Autodesk Fusion 360 part; units mm, degrees
sketch "Sketch1" plane through (0, 0, 0) normal (0, 1, 0) x (1, 0, 0)
  line L0 (0, 0) -> (250.5, 0) construction
  line L1 (250.5, 0) -> (250.5, -213.77) construction
  line L2 (250.5, -213.77) -> (0, -213.77) construction
  line L3 (0, -213.77) -> (0, 0) construction
  dimension "d1" = 250.5
  dimension "d2" = 213.77
sketch "Sketch2" plane through (0, 0, 0) normal (0, 1, 0) x (1, 0, 0)
  line L0 (0, 0) -> (250, 0) construction
  line L1 (250, 0) -> (250, -129.65) construction
  line L2 (250, -129.65) -> (0, -129.65) construction
  line L3 (0, -129.65) -> (0, 0) construction
  line L4 (193.51, 174.3203) -> (193.51, 171.7713)
  line L5 (193.51, -171.7713) -> (193.51, -174.3361)
  line L6 (169.51, 168.436) -> (169.51, 165.8296)
  line L7 (169.51, -165.8296) -> (169.51, -168.436)
  line L8 (133.51, 155.0829) -> (133.51, 152.3361)
  line L9 (133.51, -152.3361) -> (133.51, -155.0829)
  line L10 (110.01, 143.0564) -> (110.01, 140.1696)
  line L11 (110.01, -140.1696) -> (110.01, -143.0564)
  line L12 (228.8785, 178.9674) -> (228.8785, -179.12)
  arc A0 (193.51, 171.7713) -> (169.51, 165.8296) centre (246.9617, -95.5777) ccw
  arc A1 (169.51, -165.8296) -> (193.51, -171.7713) centre (246.9617, 95.5777) ccw
  arc A2 (133.51, 152.3361) -> (110.01, 140.1696) centre (246.9617, -95.5777) ccw
  arc A3 (110.01, -140.1696) -> (133.51, -152.3361) centre (246.9617, 95.5777) ccw
  arc A4 (228.8785, 178.9674) -> (193.51, 174.3203) centre (246.9617, -95.5777) ccw
  arc A5 (193.51, -174.3361) -> (228.8785, -179.12) centre (247.9959, 95.355) ccw
  arc A6 (169.51, 168.436) -> (133.51, 155.0829) centre (246.9617, -95.5777) ccw
  arc A7 (133.51, -155.0829) -> (169.51, -168.436) centre (246.9617, 95.5777) ccw
  arc A8 (110.01, 143.0564) -> (75.51, 119.6114) centre (246.9617, -95.5777) ccw
  arc A9 (75.51, -119.6114) -> (110.01, -143.0564) centre (246.9617, 95.5777) ccw
  line L13 (0, -129.65) -> (0, -95)
  line L14 (0, -95) -> (50, -95)
  line L15 (334.2254, -100.76) -> (-102.5424, -100.76) construction
  line L16 (50, -95) -> (75.51, -100.76)
  line L17 (75.51, -100.76) -> (75.51, -119.6114)
  arc A10 (72.3943, -123.5219) -> (115.01, -151.54) centre (246.9617, 95.5777) ccw
  line L18 (115.01, -148.7023) -> (115.01, -151.54)
  arc A11 (115.01, -148.7023) -> (128.51, -155.5262) centre (246.9617, 95.5777) ccw
  line L19 (128.51, -155.5262) -> (128.51, -158.2876)
  arc A12 (128.51, -158.2876) -> (174.51, -175.0312) centre (246.9617, 95.5777) ccw
  line L20 (174.51, -172.4423) -> (174.51, -175.0312)
  arc A13 (174.51, -172.4423) -> (188.51, -175.8396) centre (246.9617, 95.5777) ccw
  line L21 (188.51, -175.8396) -> (188.51, -178.3964)
  arc A14 (188.51, -178.3964) -> (228.8785, -184.1319) centre (247.9959, 95.355) ccw
  line L22 (75.51, 119.6114) -> (75.51, 0)
  line L23 (75.51, -100.76) -> (75.51, -119.6114)
  line L24 (5, -129.65) -> (5, -100)
  line L25 (5, -100) -> (49.4425, -100)
  line L26 (49.4425, -100) -> (70.51, -104.7569)
  line L27 (70.51, -104.7569) -> (70.51, -122.0073)
  arc A15 (70.51, -122.0073) -> (107.5212, -147.393) centre (246.9617, 95.5777) ccw
  line L28 (5, -129.65) -> (0, -129.65)
  line L29 (250, 0) -> (250, -213.77) construction
  line L30 (228.8785, -184.1319) -> (245, -184.1319)
  line L31 (228.8785, -179.12) -> (250, -179.12)
  line L32 (250, -179.12) -> (250, -213.77)
  line L33 (250, -213.77) -> (245, -213.77)
  line L34 (245, -213.77) -> (245, -184.1319)
  dimension "d3" = 250
  dimension "d5" = 95
  dimension "d6" = 34.65
  dimension "d7" = 50
  dimension "d8" = 100.76
  dimension "d10" = 5
  dimension "d11" = 213.77
  dimension "d12" = 34.65
  dimension "d13" = 5
revolve "Revolve1" add sketch "Sketch2" angle 360 about axis through (0, 0, 0) along (1, 0, 0)
sketch "Sketch3" plane through (0, 0, 0) normal (-1, 0, 0) x (0, -1, 0)
  circle A0 centre (0, 0) radius 129.65
  circle A1 centre (0, 0) radius 95
  line L0 (0, 0) -> (0, 238.1299) construction
  circle A2 centre (0, 122.5) radius 2
  dimension "d15" = 4
  dimension "d16" = 122.5
extrude "Extrude1" cut sketch "Sketch3" against normal blind 35 contours A2
sketch "Sketch4" plane through (250, 0, 0) normal (1, 0, 0) x (0, 1, 0)
  circle A0 centre (0, 0) radius 179.12
  circle A1 centre (0, 0) radius 213.77
  line L0 (0, 0) -> (0, 246.5899) construction
  circle A2 centre (0, 200) radius 2
  dimension "d19" = 4
  dimension "d20" = 200
extrude "Extrude2" cut sketch "Sketch4" against normal blind 27 contours A2
pattern_circular "C-Pattern1" count 20 over 360 about axis through (1.75, 0, 0) along (1, 0, 0) of "Extrude2", "Extrude1"
equation "d5 = ( 190 / 2 ) * 1 mm"
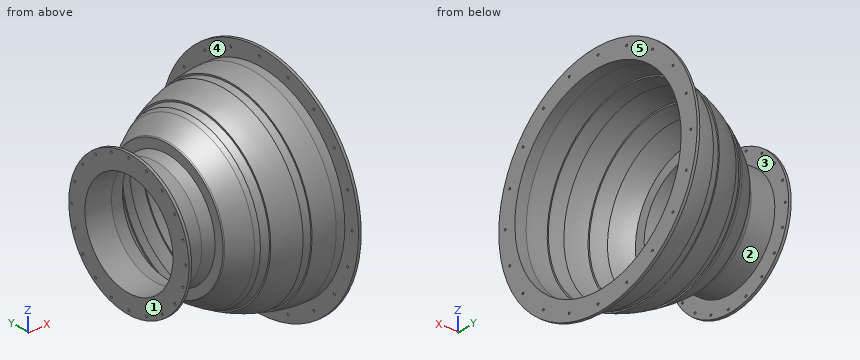
The model under review builds one solid part; all positions refer to its coordinate system, in mm. Face numbers are marked on the shaded views. A direction names the side the tool comes from. Coordinates: 2 decimals unless noted, no trailing zeros. Loops run counter-clockwise (first coordinate to the right, second up) from the corner with the lowest first, then second, coordinate; pieces in that order, holes last.
(1) Insertion check: P1, Ø8, axis at x = 200.5, z = 59.5, coming from the -Y side; P2, Ø5, axis at y = -99.1, z = 72, coming from the +X side; P3, Ø3.5, axis at y = -37.85, z = -116.5, coming from the -X side. Each pin has a flat end and moves straight along its axis. Give the tip position at first contact, or say it passes through.
Determined:
P1: stops at y = -172.18
P2: stops at x = 82.49
P3: stops at x = 70.51
(2) Draft analysis for pull direction X (two halves, no side actions). For the marked faces 3, 4 and 5, state which applies: +X half, -X half, draft (parallel to the pull), parting line (faces both ways), or undercut.
Determined:
face 3: undercut
face 4: -X half
face 5: +X half
(3) Consider section A-A, the plane x = 39.5. Give the boundary of the cut face in (y, z).
Determined:
outline: circle Ø200 at (0, 0); hole circle Ø190 at (0, 0)
(4) Wall thickness on L1, parallel to Z at x = 247.75, y = 0; L2, parallel to Z at x = 172, y = 113.5: over which ranges is each line inside the solid? List them lowest first.
Determined:
L1: z = -213.77 to -202, -198 to -179.12, 179.12 to 198, 202 to 213.77
L2: z = -132.34 to -121.89, 121.89 to 132.34
(5) Tool access review of the marked faces 1 and 2: name each direction out of +Z, -Z, +X, -X, +Y, -Y from which nothing blocks a thin tool from reaching the whole face with its end or side.
Determined:
face 1: +Z, -Z, -X, +Y, -Y
face 2: none
